Could you check a few things on this model? Use its own coordinates, in mm. A direction names the side the tool comes from. Coordinates: 2 decimals unless noted, no trailing zeros. Order: outer loops, then holes, each group sorted by start corner. A loop starts at its lowest first (then second) coordinate and runs counter-clockwise, first axis right, second up. Notation, with made-up numbers: (27, 75.25) -> (46, 75.25) arc R31 cw to (46, 109.25) -> close; hole circle Ø4 at (1, 10). An arc over 180 degrees is marked (long way). Put each result on its own line as item: value. Start each with the question number.
Q1. Will this pin go through, and if not, where does the flat tip stop? pin 1 (1.5 mm diameter, centred on x = 34.5, y = -85.78, fed in from -Z).
Q2. For faces 5 (the face through (29, -52, 2)), 6 (the face through (30, -50, 0)), which set-ups out of +Z, -Z, +X, -X, +Y, -Y let a thin tool reach every point of the face, with its end or its side?
Q3. If we section it at C-C (x = 28): Please give me the cut outline in (y, z).
Q4. Please list where these lines run through material, in increasing order: line 1 along Y through (x, z) = (34.5, 0.7); line 2 along X through (y, z) = (-28.5, 2.25); line 3 along Y through (x, z) = (21.5, 0.7).
Q5. If we section it at A-A (x = 34.5): Please give me the cut outline in (y, z), and give its area (3 significant figures).
Q6. We'd pull the mould along Y, two halves only. Please class faces 1 (the face through (0, -52, 1)), 2 (the face through (35.13, -85.21, 1.48)), 3 (the face through (18, -96.003, 1)), 4 (the face through (35.35, -16.19, 1.48)): +Y half, -Y half, draft (parallel to the pull), parting line (faces both ways), or undercut.
Q7. If we section it at D-D (z = 2.4): Please give me the cut outline in (x, y).
Q8. If we section it at B-B (y = -20): Please give me the cut outline in (x, z).
from build123d import *

# Parameters (mm, degrees)
SKETCH1_W           = 36
SKETCH1_H           = 90
SKETCH1_W_2         = 30
SKETCH1_H_2         = 67
BOSS_EXTRUDE1_DEPTH = 3
SKETCH3_R           = 0.85
CUT_EXTRUDE1_DEPTH  = 3
SKETCH4_W           = 4
SKETCH4_H           = 67
BOSS_EXTRUDE2_DEPTH = 3


with BuildPart() as part:
    # Sketch1 → Boss-Extrude1 (new body)
    with BuildSketch(Plane.XY):
        with Locations((18, -51.003070917)):
            Rectangle(SKETCH1_W, SKETCH1_H)
        with Locations((18, -51.503070917)):
            Rectangle(SKETCH1_W_2, SKETCH1_H_2, mode=Mode.SUBTRACT)
    extrude(amount=BOSS_EXTRUDE1_DEPTH)

    # Sketch3 → Cut-Extrude1 (cut)
    with BuildSketch(Plane(origin=(0, 0, 0), x_dir=(-1, 0, 0), z_dir=(0, 0, -1))):
        with Locations((-34.5, -16.224619538)):
            Circle(SKETCH3_R)
        with Locations((-1.5, -16.224619538)):
            Circle(SKETCH3_R)
        with Locations((-1.5, -85.781522297)):
            Circle(SKETCH3_R)
        with Locations((-34.5, -85.781522297)):
            Circle(SKETCH3_R)
    extrude(amount=-CUT_EXTRUDE1_DEPTH, mode=Mode.SUBTRACT)

    # Sketch4 → Boss-Extrude2 (add)
    with BuildSketch(Plane.XY.offset(3)):
        with Locations((31, -51.503070917)):
            Rectangle(SKETCH4_W, SKETCH4_H)
    extrude(amount=-BOSS_EXTRUDE2_DEPTH)


solid = part.part
The answers:
1. pin 1: through
2. face 5: +Z, -Z
2. face 6: -Z, +X, -X, +Y, -Y
3. outline: (-96, 0) -> (-85, 0) -> (-85, 3) -> (-96, 3) -> close; (-18, 0) -> (-6, 0) -> (-6, 3) -> (-18, 3) -> close
4. line 1: -96 to -86.63, -84.93 to -17.07, -15.37 to -6
4. line 2: 0 to 3, 29 to 36
4. line 3: -96 to -85, -18 to -6
5. outline: (-96, 0) -> (-86.63, 0) -> (-86.63, 3) -> (-96, 3) -> close; (-84.93, 0) -> (-17.07, 0) -> (-17.07, 3) -> (-84.93, 3) -> close; (-15.37, 0) -> (-6, 0) -> (-6, 3) -> (-15.37, 3) -> close
5. area: 260 mm^2
6. face 1: draft
6. face 2: undercut
6. face 3: -Y half
6. face 4: undercut
7. outline: (0, -96) -> (36, -96) -> (36, -6) -> (0, -6) -> close; hole circle Ø1.7 at (1.5, -85.78); hole circle Ø1.7 at (1.5, -16.22); hole (3, -85) -> (29, -85) -> (29, -18) -> (3, -18) -> close; hole circle Ø1.7 at (34.5, -85.78); hole circle Ø1.7 at (34.5, -16.22)
8. outline: (0, 0) -> (3, 0) -> (3, 3) -> (0, 3) -> close; (29, 0) -> (36, 0) -> (36, 3) -> (29, 3) -> close
